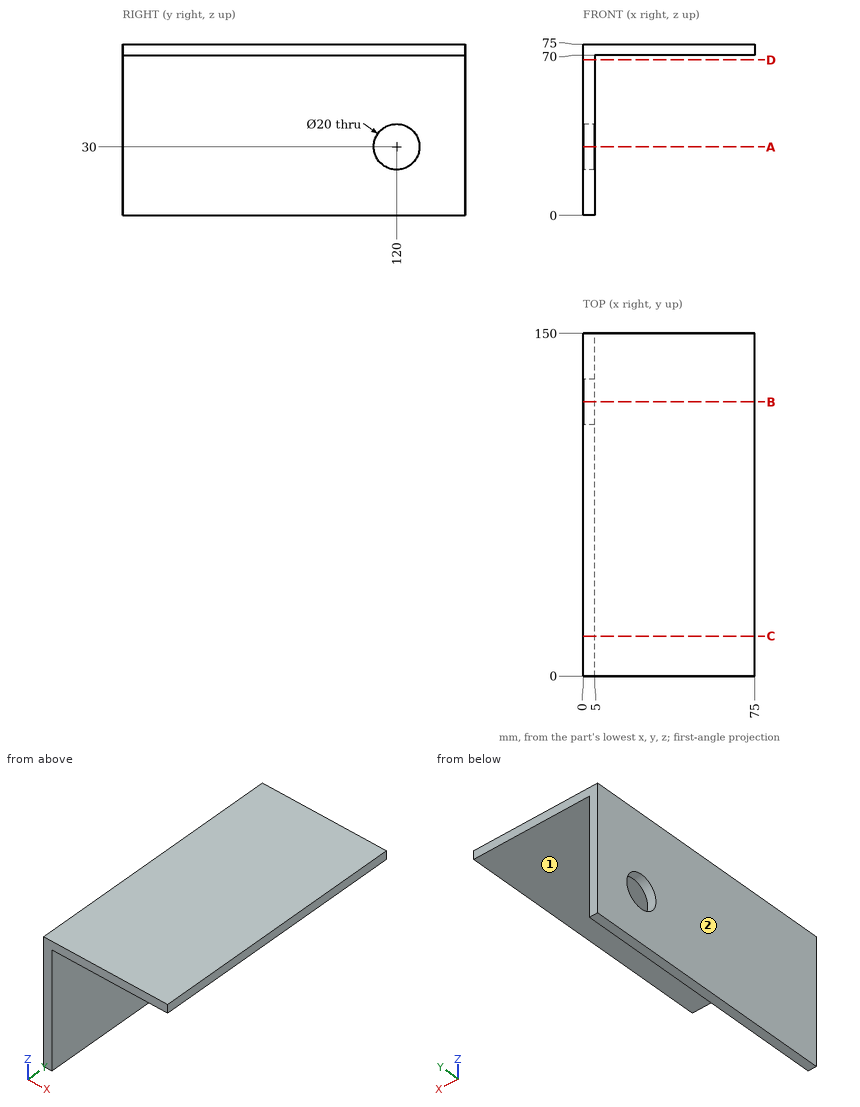
Geometry check sheet. Reference: drawing and pictorial views, mm from the part's lowest x, y, z. A direction names the side the tool comes from. Round coordinates to 2 decimals unless told otherwise and drop trailing zeros. Order: outer loops, then holes, each group sorted by start corner. A loop starts at its lowest first (then second) coordinate and runs counter-clockwise, first axis right, second up. Notation, with made-up numbers: (7, 70) - (35, 70) arc R13 ccw to (35, 85) - close; hole circle Ø8 at (16.5, -4). An arc over 180 degrees is marked (long way). Use a Markdown table: item, result. Add a question column.
1) Set-up check for the marked faces 1 and 2: record each of +Z, -Z, +X, -X, +Y, -Y from which the full face is reachable in a straight line by a thin tool's end or side.
2) Gauge pin test, flat ends, axial feed: P1, Ø1, axis at y = 89, z = 56, coming from the +X side; P2, Ø4, axis at x = 10, y = 52, coming from the -Z side. Record the tip position at first contact, or that the pin passes through.
3) Section check D-D (z = 68). Record the cut outline in (x, y).
4) Section check B-B (y = 120). Record the cut outline in (x, z), then the cut area to 3 significant figures.
5) Section check C-C (y = 17.5). Record the cut outline in (x, z).
6) Section check A-A (z = 30). Record the cut outline in (x, y), then the cut area to 3 significant figures.
7) Thickness scan on line 1 along Y through (x, z) = (1.2, 30); line 2 along X through (y, z) = (127.5, 6); line 3 along Z through (x, y) = (26.5, 70.5). Record the ranges inside material, lowest first.
Established:
| question | item | result |
|---|---|---|
| 1 | face 1 | -Z, +X, +Y, -Y |
| 1 | face 2 | +Z, -Z, -X, +Y, -Y |
| 2 | P1 | x = 5 |
| 2 | P2 | z = 70 |
| 3 | outline | (0, 0) - (5, 0) - (5, 150) - (0, 150) - close |
| 4 | outline | (0, 0) - (5, 0) - (5, 20) - (0, 20) - close; (0, 40) - (5, 40) - (5, 70) - (75, 70) - (75, 75) - (0, 75) - close |
| 4 | area | 625 mm2 |
| 5 | outline | (0, 0) - (5, 0) - (5, 70) - (75, 70) - (75, 75) - (0, 75) - close |
| 6 | outline | (0, 0) - (5, 0) - (5, 110) - (0, 110) - close; (0, 130) - (5, 130) - (5, 150) - (0, 150) - close |
| 6 | area | 650 mm2 |
| 7 | line 1 | 0 to 110, 130 to 150 |
| 7 | line 2 | 0 to 5 |
| 7 | line 3 | 70 to 75 |
